Part model, mm, in its own coordinate system. Give positions to 0.01 mm unless a question says otherwise; leave off trailing zeros. Write each loop counter-clockwise with the first axis right and the second up, starting at its lowest first coordinate (ties: lowest second). Pieces come first, ordered by that corner, then holes.
```python
from build123d import *

# Parameters (mm, degrees)
F1_DEPTH = 1.25


with BuildPart() as f1:
    # F0 (on Top) → F1 (new body)
    with BuildSketch(Plane.XY):
        with BuildLine():
            Line((-1.375, -2.25), (1.375, -2.25))
            ThreePointArc((1.375, -2.25), (3.625, 0), (1.375, 2.25))
            Line((1.375, 2.25), (-1.375, 2.25))
            ThreePointArc((-1.375, 2.25), (-3.625, 0), (-1.375, -2.25))
        make_face()
    extrude(amount=F1_DEPTH)

    # F2 (on Front) → F3 (revolve)
    with BuildSketch(Plane.XZ):
        with BuildLine():
            Line((-1.5, 1.25), (0, 1.25))
            Line((0, 1.25), (0, 5.75))
            Line((0, 5.75), (-0.552479, 5.75))
            ThreePointArc((-0.552479, 5.75), (-0.885939, 5.622564), (-1.04942, 5.305216))
            Line((-1.04942, 5.305216), (-1.5, 1.25))
        make_face()
    revolve(axis=Axis((0, 0, 3.5), (0, 0, 1)))


solid = f1.part
```
1) Saw through at A-A, the plane y = 0. Write the cut outline in (x, z) (3 decimals).
Answers follow:
outline: (-3.625, 0) - (3.625, 0) - (3.625, 1.25) - (1.5, 1.25) - (1.049, 5.305) arc R0.5 ccw to (0.552, 5.75) - (-0.552, 5.75) arc R0.5 ccw to (-1.049, 5.305) - (-1.5, 1.25) - (-3.625, 1.25) - close
2) Saw through at B-B, the plane x = 0. Write the cut outline in (y, z), then the cut area to 3 significant figures.
Answers follow:
outline: (-2.25, 0) - (2.25, 0) - (2.25, 1.25) - (1.5, 1.25) - (1.05, 5.31) arc R0.5 ccw to (0.55, 5.75) - (-0.55, 5.75) arc R0.5 ccw to (-1.05, 5.31) - (-1.5, 1.25) - (-2.25, 1.25) - close
area: 16.8 mm2
3) Pin check, flat tips, straight feed: pin 1 Ø2 at (y, z) = (1.5, 4.5) entering from -X; pin 2 Ø1.5 at (y, z) = (-1, 1) entering from +X. Stop position of each tip, or through.
Answers follow:
pin 1: stops at x = -1.04
pin 2: stops at x = 3.61
4) Wall check: L1, parallel to Z at x = 2.5, y = 0.35; L2, parallel to X at y = 0.5, z = 5.45; L3, parallel to X at y = 0.5, z = 4.6. Give the ranges that are in metal, low to high.
Answers follow:
L1: z = 0 to 1.25
L2: x = -0.88 to 0.88
L3: x = -1.01 to 1.01
5) Saw through at D-D, the plane y = -1.6. Write the cut outline in (x, z), then the cut area to 3 significant figures.
Answers follow:
outline: (-2.96, 0) - (2.96, 0) - (2.96, 1.25) - (-2.96, 1.25) - close
area: 7.39 mm2
6) Saw through at C-C, the plane z = 2. Write the cut outline in (x, y).
Answers follow:
outline: circle Ø2.83 at (0, 0)
